The model under review builds one solid part; all positions refer to its coordinate system, in mm. Round coordinates to 2 decimals unless told otherwise and drop trailing zeros. Order: outer loops, then holes, each group sorted by start corner. A loop starts at its lowest first (then second) coordinate and runs counter-clockwise, first axis right, second up. Notation, with made-up numbers: (62.25, 33) - (91.25, 33) arc R28 cw to (91.25, 51) - close; hole circle Ø1 at (13.25, -24). An arc over 180 degrees is marked (long way). One line per question, with ' | ' between items. Start each with the question number.
Item 1: Draft analysis for pull direction X (two halves, no side actions). For faces 1 (the face through (0, -30, 6)), 2 (the face through (39.07, 38.71, 5.92)), 3 (the face through (-2.38, -10.74, 5.92)), 4 (the face through (-38.71, 39.07, 5.92)), state which applies: +X half, -X half, draft (parallel to the pull), parting line (faces both ways), or undercut.
Item 2: Add section A-A on x = 0. State the section outline as (y, z) points, and give its area (3 significant figures).
Item 3: Add section B-B on z = 6.5. State the section outline as (x, y) points, and give its area (3 significant figures).
Item 4: Insertion check: pin 1 Ø1 at (x, z) = (-34, 2) entering from +Y; pin 2 Ø1.5 at (y, z) = (39.5, 7) entering from +X; pin 3 Ø2 at (x, z) = (-27.5, 8) entering from -Y. Each pin has a flat end and moves straight along its axis. Give the tip position at first contact, or say it passes through.
Item 5: For L1, parallel to Y at x = -4.5, z = 4.75; L2, parallel to Y at x = -32.5, z = 8.5; L3, parallel to X at y = 9.5, z = 3.5, list the stretches that pass through material, from the lowest coordinate up. Write a range as [from, to].
Item 6: Add section C-C on x = 41.5. State the section outline as (y, z) points, and give its area (3 significant figures).
Item 7: Add section D-D on y = -28. State the section outline as (x, z) points, and give its area (3 significant figures).
from build123d import *

# Parameters (mm, degrees)
F0_R     = 11
F1_DEPTH = 12


with BuildPart() as f1:
    # F0 (on Top) → F1 (new body)
    with BuildSketch(Plane.XY):
        with BuildLine():
            ThreePointArc((49.318182, -24.345779), (30, 0), (49.318182, 24.345779))
            ThreePointArc((49.318182, 24.345779), (38.890873, 38.890873), (24.345779, 49.318182))
            ThreePointArc((24.345779, 49.318182), (0, 30), (-24.345779, 49.318182))
            ThreePointArc((-24.345779, 49.318182), (-38.890873, 38.890873), (-49.318182, 24.345779))
            ThreePointArc((-49.318182, 24.345779), (-35.416264, 15.539539), (-30, 0))
            ThreePointArc((-30, 0), (-35.416264, -15.539539), (-49.318182, -24.345779))
            ThreePointArc((-49.318182, -24.345779), (-38.890873, -38.890873), (-24.345779, -49.318182))
            ThreePointArc((-24.345779, -49.318182), (0, -30), (24.345779, -49.318182))
            ThreePointArc((24.345779, -49.318182), (38.890873, -38.890873), (49.318182, -24.345779))
        make_face()
        Circle(F0_R, mode=Mode.SUBTRACT)
    extrude(amount=F1_DEPTH)


solid = f1.part
Determined:
1) face 1: undercut | face 2: +X half | face 3: undercut | face 4: -X half
2) outline: (-30, 0) - (-11, 0) - (-11, 12) - (-30, 12) - close; (11, 0) - (30, 0) - (30, 12) - (11, 12) - close | area: 456 mm2
3) outline: (-49.32, -24.35) arc R55 ccw to (-24.35, -49.32) arc R25 cw to (24.35, -49.32) arc R55 ccw to (49.32, -24.35) arc R25 cw to (49.32, 24.35) arc R55 ccw to (24.35, 49.32) arc R25 cw to (-24.35, 49.32) arc R55 ccw to (-49.32, 24.35) arc R25 cw to (-30, 0) arc R25 cw to start; hole circle Ø22 at (0, 0) | area: 5,580 mm2
4) pin 1: y = 43.62 | pin 2: x = 39.03 | pin 3: y = -48.19
5) L1: [-30.41, -10.04], [10.04, 30.41] | L2: [-44.37, -10.9], [10.9, 44.37] | L3: [-31.88, -5.55], [5.55, 31.88]
6) outline: (-36.09, 0) - (-21.04, 0) - (-21.04, 12) - (-36.09, 12) - close; (21.04, 0) - (36.09, 0) - (36.09, 12) - (21.04, 12) - close | area: 361 mm2
7) outline: (-47.34, 0) - (47.34, 0) - (47.34, 12) - (-47.34, 12) - close | area: 1,140 mm2
